Source: CAD feature listing. Evaluate the final solid. Frame: model axes, mm. A direction names the side the tool comes from. Round coordinates to 2 decimals unless told otherwise and drop trailing zeros. Order: outer loops, then holes, each group sorted by start corner. A loop starts at its lowest first (then second) coordinate and runs counter-clockwise, first axis right, second up. Notation, with made-up numbers: (2.5, 33) - (56.5, 33) arc R7 cw to (56.5, 46) - close; hole circle Ø2 at (-0.75, 80). An arc over 180 degrees is marked (long way). Put each result on its own line as item: value. Start each with the question number.
1) Section B-B on y = 111. Output: boundary loops of the cut face in (x, z).
2) Section A-A on z = 4. Output: boundary loops of the cut face in (x, y).
3) Access query for faces 4 (the face through (0, 99, 9)), 5 (the face through (-9.493, 187.804, 0.488)). Directions: +Z, -Z, +X, -X, +Y, -Y. A direction counts if a zero-diameter tool reaches every point of the face in a straight line with its end or side. Return the directions, or none.
4) Mould query, pull axis Y, two halves, no side actions, for faces 1 (the face through (1.21, 11.897, 9.507)), 2 (the face through (-0.8, 0, 9.6)), 3 (the face through (-0.8, 200, 9.6)). Classes: +Y half, -Y half, draft (parallel to the pull), parting line (faces both ways), or undercut.
5) Contact query for flat-ended pins moving along their axis: P1, Ø7, axis at x = 0, y = 20, coming from the +Z side; P2, Ø3.5, axis at x = 0, y = 10, coming from the -Z side. Output: stop coordinate, or through.
6) Line query: probe 1 along X at (y, z) = (25.5, 8); probe 2 along Y at (x, z) = (9.5, 0). Output: solid intervals per line, ascending. Write a range as [from, to].
7) Section D-D on x = 0. State how many separate pieces and enclosed holes the cut face has, then the cut area to 3 significant figures.
8) Section C-C on y = 40. Output: boundary loops of the cut face in (x, z).
```python
from build123d import *

# Parameters (mm, degrees)
SKETCH1_W           = 20
SKETCH1_H           = 20
SKETCH1_W_2         = 18
SKETCH1_H_2         = 18
BOSS_EXTRUDE1_DEPTH = 200
SKETCH2_R           = 2.25
CUT_EXTRUDE1_DEPTH  = 202.246117975
SKETCH3_R           = 2.25
CUT_EXTRUDE2_DEPTH  = 202.246117975


with BuildPart() as part:
    # Sketch1 → Boss-Extrude1 (new body)
    with BuildSketch(Plane(origin=(0, 0, 0), x_dir=(1, 0, 0), z_dir=(0, 1, 0))):
        Rectangle(SKETCH1_W, SKETCH1_H)
        Rectangle(SKETCH1_W_2, SKETCH1_H_2, mode=Mode.SUBTRACT)
    extrude(amount=BOSS_EXTRUDE1_DEPTH)

    # Sketch2 → Cut-Extrude1 (cut, through all)
    with BuildSketch(Plane.XY.offset(10)):
        with Locations((0, 10)):
            Circle(SKETCH2_R)
        with Locations((0, 20)):
            Circle(SKETCH2_R)
        with Locations((0, 30)):
            Circle(SKETCH2_R)
        with Locations((0, 40)):
            Circle(SKETCH2_R)
        with Locations((0, 50)):
            Circle(SKETCH2_R)
        with Locations((0, 60)):
            Circle(SKETCH2_R)
    extrude(amount=-CUT_EXTRUDE1_DEPTH, mode=Mode.SUBTRACT)

    # Sketch3 → Cut-Extrude2 (cut, through all)
    with BuildSketch(Plane(origin=(10, 0, 0), x_dir=(0, 0, -1), z_dir=(1, 0, 0))):
        with Locations((0, 190)):
            Circle(SKETCH3_R)
    extrude(amount=-CUT_EXTRUDE2_DEPTH, mode=Mode.SUBTRACT)


solid = part.part
```
Answer sheet:
1. outline: (-10, -10) - (10, -10) - (10, 10) - (-10, 10) - close; hole (-9, -9) - (9, -9) - (9, 9) - (-9, 9) - close
2. outline: (-10, 0) - (-9, 0) - (-9, 200) - (-10, 200) - close; (9, 0) - (10, 0) - (10, 200) - (9, 200) - close
3. face 4: +Y, -Y
3. face 5: +X, -X
4. face 1: undercut
4. face 2: -Y half
4. face 3: +Y half
5. P1: z = 10
5. P2: through
6. probe 1: [-10, -9], [9, 10]
6. probe 2: [0, 187.75], [192.25, 200]
7. separate pieces: 14
7. enclosed holes: 0
7. area: 346 mm^2
8. outline: (-10, -10) - (-2.25, -10) - (-2.25, -9) - (-9, -9) - (-9, 9) - (-2.25, 9) - (-2.25, 10) - (-10, 10) - close; (2.25, -10) - (10, -10) - (10, 10) - (2.25, 10) - (2.25, 9) - (9, 9) - (9, -9) - (2.25, -9) - close
